from build123d import *

# Parameters (mm, degrees)
SKETCH1_R                                      = 38.1
BOSS_EXTRUDE1_DEPTH                            = 6.35
CBORE_FOR_4_BUTTON_HEAD_CAP_SCREW1_D           = 2.9464
CBORE_FOR_4_BUTTON_HEAD_CAP_SCREW1_CBORE_D     = 5.715
CBORE_FOR_4_BUTTON_HEAD_CAP_SCREW1_CBORE_DEPTH = 1.4986
CIRPATTERN1_COUNT                              = 8
SKETCH8_R                                      = 4.7625
CUT_EXTRUDE1_DEPTH                             = 55.254423783


with BuildPart() as part:
    # Sketch1 → Boss-Extrude1 (new body)
    with BuildSketch(Plane(origin=(0, 0, 0), x_dir=(1, 0, 0), z_dir=(0, 1, 0))):
        with Locations(Location((0, 0, 0), (0, 0, 270))):
            Circle(SKETCH1_R)
    extrude(amount=BOSS_EXTRUDE1_DEPTH)

    # CBORE for #4 Button Head Cap Screw1 (through all)
    with Locations(Plane(origin=(0, 0, 0), x_dir=(-1, 0, 0), z_dir=(0, -1, 0))):
        with Locations((0, -33.3375)):
            cbore_for_4_button_head_cap_screw1 = CounterBoreHole(CBORE_FOR_4_BUTTON_HEAD_CAP_SCREW1_D / 2, CBORE_FOR_4_BUTTON_HEAD_CAP_SCREW1_CBORE_D / 2, CBORE_FOR_4_BUTTON_HEAD_CAP_SCREW1_CBORE_DEPTH)

    # CirPattern1: CBORE for #4 Button Head Cap Screw1 ×8 about axis
    cirpattern1_axis = Axis((0, 0, 0), (0, 1, 0))
    for i in range(1, CIRPATTERN1_COUNT):
        add(cbore_for_4_button_head_cap_screw1.rotate(cirpattern1_axis, i * 360 / CIRPATTERN1_COUNT), mode=Mode.SUBTRACT)

    # Sketch8 → Cut-Extrude1 (cut, through all)
    with BuildSketch(Plane.XZ):
        with Locations(Location((0, 0, 0), (0, 0, 270))):
            Circle(SKETCH8_R)
    extrude(amount=-CUT_EXTRUDE1_DEPTH, mode=Mode.SUBTRACT)


solid = part.part
Geometry check sheet. Reference: the model listing, model coordinates, mm. A direction names the side the tool comes from. Round coordinates to 2 decimals unless told otherwise and drop trailing zeros. Write each loop counter-clockwise with the first axis right and the second up, starting at its lowest first coordinate (ties: lowest second). Pieces come first, ordered by that corner, then holes. Notation, with made-up numbers: (79, 83) - (133, 83) arc R28 ccw to (133, 115) - close; hole circle Ø3 at (89.25, 69). An arc over 180 degrees is marked (long way). One line per item, written item: value.
1. Depth check by flat-ended pin: pin 1 Ø5 at (x, z) = (0, 33.34) entering from -Y; pin 2 Ø2.5 at (x, z) = (23.57, 23.57) entering from +Y; pin 3 Ø1.5 at (y, z) = (4, 7) entering from -X; pin 4 Ø2 at (y, z) = (3, -1) entering from -X. Enter the tip coordinate at first touch or a pass-through.
The answers:
pin 1: stops at y = 1.5
pin 2: passes through
pin 3: stops at x = -37.58
pin 4: stops at x = -38.1
2. Set-up check for faces 4 (the face through (-23.255, 3.958, -22.135)), 5 (the face through (23, 1.499, 22)): record each of +Z, -Z, +X, -X, +Y, -Y from which the full face is reachable in a straight line by a thin tool's end or side.
The answers:
face 4: +Y, -Y
face 5: -Y
3. Cross-section at A-A on z = 0. Give the number of separate pieces and of enclosed holes in the cut face, and give its area (3 significant figures).
The answers:
separate pieces: 4
enclosed holes: 0
area: 378 mm^2
4. Scan lines: L1, parallel to X at y = 3.25, z = 0; L2, parallel to X at y = 1, z = 0 (1 decimal); L3, parallel to Z at x = 3.5, y = 6.25. Record each from-to range of solid material in increasing order.
The answers:
L1: x = -38.1 to -34.81, -31.86 to -4.76, 4.76 to 31.86, 34.81 to 38.1
L2: x = -38.1 to -36.2, -30.5 to -4.8, 4.8 to 30.5, 36.2 to 38.1
L3: z = -37.94 to -3.23, 3.23 to 37.94
5. Cross-section at D-D on x = 13.5. Record the boundary of the cut face in (y, z).
The answers:
outline: (0, -35.63) - (6.35, -35.63) - (6.35, 35.63) - (0, 35.63) - close
6. Mould release check, pull along X, two halves, no side actions. Record for faces 1 (the face through (-36.127, 0.739, 0.619)), 2 (the face through (-23.183, 3.131, -30.235)), 3 (the face through (1, 6.35, 8)): released by +X, released by -X, zero draft, split by the parting line, or undercut.
The answers:
face 1: undercut
face 2: split by the parting line
face 3: zero draft
